Check sheet for the modelled part. Datum: model origin and axes. Units: mm. A direction names the side the tool comes from. Give positions to 0.01 mm unless a question says otherwise; leave off trailing zeros. Order: outer loops, then holes, each group sorted by start corner. A loop starts at its lowest first (then second) coordinate and runs counter-clockwise, first axis right, second up. Notation, with made-up numbers: (-14.75, -14) - (-3.75, -14) arc R28 ccw to (-3.75, 4) - close; hole circle Ø10 at (77.25, -27.75). An arc over 180 degrees is marked (long way). Answer in a Markdown table with one row per item.
from build123d import *

# Parameters (mm, degrees)
SKETCH1_W           = 456
SKETCH1_H           = 249
SKETCH1_W_2         = 438
SKETCH1_H_2         = 231
BOSS_EXTRUDE4_DEPTH = 9
SKETCH1_5_W         = 456
SKETCH1_5_H         = 249
SKETCH1_5_W_2       = 438
SKETCH1_5_H_2       = 231
BOSS_EXTRUDE5_DEPTH = 65
SKETCH5_W           = 231
SKETCH5_H           = 56
SKETCH5_H_2         = 9
CUT_EXTRUDE1_DEPTH  = 469.544821762
SKETCH6_W           = 4
SKETCH6_H           = 231
BOSS_EXTRUDE6_DEPTH = 65
BOSS_EXTRUDE7_START = -9
SKETCH5_3_W         = 231
SKETCH5_3_H         = 9
BOSS_EXTRUDE7_DEPTH = 21
SKETCH7_R           = 3.5
SKETCH7_R_2         = 6.4
SKETCH7_R_3         = 5.96
SKETCH7_W           = 45.5
SKETCH7_H           = 25.5
CUT_EXTRUDE2_DEPTH  = 150


with BuildPart() as part:
    # Sketch1 → Boss-Extrude4 (new body)
    with BuildSketch(Plane(origin=(0, 0, 0), x_dir=(1, 0, 0), z_dir=(0, 1, 0))):
        Rectangle(SKETCH1_W, SKETCH1_H)
        Rectangle(SKETCH1_W_2, SKETCH1_H_2, mode=Mode.SUBTRACT)
        Rectangle(SKETCH1_W_2, SKETCH1_H_2)
    extrude(amount=BOSS_EXTRUDE4_DEPTH)

    # Sketch1<5> → Boss-Extrude5 (add)
    with BuildSketch(Plane(origin=(0, 0, 0), x_dir=(1, 0, 0), z_dir=(0, 1, 0))):
        Rectangle(SKETCH1_5_W, SKETCH1_5_H)
        Rectangle(SKETCH1_5_W_2, SKETCH1_5_H_2, mode=Mode.SUBTRACT)
    extrude(amount=-BOSS_EXTRUDE5_DEPTH)

    # Sketch5 → Cut-Extrude1 (cut, through all)
    with BuildSketch(Plane.ZY.offset(-219)):
        with Locations((0, -28)):
            Rectangle(SKETCH5_W, SKETCH5_H)
        with Locations((0, -60.5)):
            Rectangle(SKETCH5_W, SKETCH5_H_2)
    extrude(amount=-CUT_EXTRUDE1_DEPTH, mode=Mode.SUBTRACT)

    # Sketch6 → Boss-Extrude6 (add)
    with BuildSketch(Plane.XZ):
        with Locations((205, 0)):
            Rectangle(SKETCH6_W, SKETCH6_H)
    extrude(amount=BOSS_EXTRUDE6_DEPTH)

    # Sketch5<3> → Boss-Extrude7 (add)
    with BuildSketch(Plane.ZY.offset(-219).offset(BOSS_EXTRUDE7_START)):
        with Locations((0, -60.5)):
            Rectangle(SKETCH5_3_W, SKETCH5_3_H)
    extrude(amount=BOSS_EXTRUDE7_DEPTH)

    # Sketch7 → Cut-Extrude2 (cut)
    with BuildSketch(Plane(origin=(207, 0, 0), x_dir=(0, 0, -1), z_dir=(1, 0, 0))):
        with Locations((-90.5, -28)):
            Circle(SKETCH7_R)
        with Locations((66.4, -28)):
            Circle(SKETCH7_R_2)
        with Locations((93.76, -28)):
            Circle(SKETCH7_R_3)
        with Locations((22.25, -28)):
            Rectangle(SKETCH7_W, SKETCH7_H)
    extrude(amount=-CUT_EXTRUDE2_DEPTH, mode=Mode.SUBTRACT)


solid = part.part
(1) Gauge pin test, flat ends, axial feed: P1, Ø3, axis at x = -141, z = 44.5, coming from the -Y side; P2, Ø4, axis at y = -28, z = 90.5, coming from the +X side. Record the tip position at first contact, or that the pin passes through.
Geometry says:
| item | result |
|---|---|
| P1 | y = 0 |
| P2 | x = -219 |
(2) Cross-section at A-A, the plane z = -93.76. Record the cut outline in (x, y), then the cut area to 3 significant figures.
Geometry says:
| item | result |
|---|---|
| outline | (-228, -65) - (-219, -65) - (-219, 0) - (203, 0) - (203, -22.04) - (207, -22.04) - (207, 0) - (228, 0) - (228, 9) - (-228, 9) - close; (203, -65) - (228, -65) - (228, -56) - (207, -56) - (207, -33.96) - (203, -33.96) - close |
| area | 5,090 mm² |
(3) Mould release check, pull along Y, two halves, no side actions. Record for faces 1 (the flat face through (218, -56, -2)), 2 (the flat face through (-3, -27, 124.5)), 3 (the flat face through (-3, 9, -2)): pulls with the +Y half, pulls with the -Y half, needs draft (parallel to the pull), parting line crosses it, or undercut.
Geometry says:
| item | result |
|---|---|
| face 1 | undercut |
| face 2 | needs draft |
| face 3 | pulls with the +Y half |
(4) Cross-section at D-D, the plane z = 27. Record the cut outline in (x, y).
Geometry says:
| item | result |
|---|---|
| outline | (-228, -65) - (-219, -65) - (-219, 0) - (203, 0) - (203, -65) - (228, -65) - (228, -56) - (207, -56) - (207, 0) - (228, 0) - (228, 9) - (-228, 9) - close |
(5) Cross-section at C-C, the plane x = 149.5. Record the cut outline in (y, z), then the cut area to 3 significant figures.
Geometry says:
| item | result |
|---|---|
| outline | (-65, -124.5) - (9, -124.5) - (9, 124.5) - (-65, 124.5) - (-65, 115.5) - (0, 115.5) - (0, -115.5) - (-65, -115.5) - close |
| area | 3,410 mm² |
(6) Thickness scan on L1, parallel to Z at x = -190.5, y = -39.5; L2, parallel to X at y = -51, z = 27; L3, parallel to Y at x = 205.4, z = 90.5. Record the ranges inside material, lowest first.
Geometry says:
| item | result |
|---|---|
| L1 | -124.5 to -115.5, 115.5 to 124.5 |
| L2 | -228 to -219, 203 to 207 |
| L3 | -65 to -31.5, -24.5 to 9 |
(7) Access from +Z, -Z, +X, -X, +Y, -Y to the whole of each face (thin tool, end or side, straight path). Record for faces 4 (the flat face through (203, -46, -2)), 5 (the flat face through (217, 0, -2)), 6 (the flat face through (228, -58, -10)).
Geometry says:
| item | result |
|---|---|
| face 4 | -Y |
| face 5 | +X |
| face 6 | +Z, -Z, +X, +Y, -Y |
(8) Cross-section at B-B, the plane y = -9. Record the cut outline in (x, z).
Geometry says:
| item | result |
|---|---|
| outline | (-228, -124.5) - (228, -124.5) - (228, -115.5) - (207, -115.5) - (207, 115.5) - (228, 115.5) - (228, 124.5) - (-228, 124.5) - close; hole (-219, -115.5) - (203, -115.5) - (203, 115.5) - (-219, 115.5) - close |
